Read the model definition and answer for the solid it produces. Units are mm, in the model's axes. A direction names the side the tool comes from. Coordinates: 2 decimals unless noted, no trailing zeros. Write each loop counter-clockwise with the first axis right and the second up, starting at its lowest first coordinate (ties: lowest second). Pieces come first, ordered by that corner, then holes.
(1) The mould has two halves that part along Y. Classify faces 1 (the conical face through (-23.226, 19.757, -0.871)), 2 (the cylindrical face through (-11.668, 34.51, -15.217)), 3 (the flat face through (69, 0, 0)), 4 (the conical face through (163.226, 50.243, 0.871)): +Y half, -Y half, draft (parallel to the pull), parting line (faces both ways), or undercut.
(2) Section A-A on z = 0 is taken. Write down the section's boundary in (x, y) (3 decimals), then the cut area to 3 significant figures.
(3) Which of the six approach directions +Z, -Z, +X, -X, +Y, -Y give full straight-line access (tool end or side, diameter ignored) to faces 5 (the conical face through (163.226, 19.757, 0.871)), 6 (the cylindrical face through (121.28, 34.51, -4.16))?
(4) Find the intervals of material crossed by probe 1 along X at (y, z) = (32, 0) (3 decimals); probe 2 along X at (y, z) = (34.5, -6); probe 3 along X at (y, z) = (32.5, -17.5), in increasing order.
(5) Section C-C on x = 80 is taken. Write down the section's boundary in (y, z), then the cut area to 3 significant figures.
(6) Given pin 1 (2 mm diameter, centred on y = 21, z = 16.5, fed in from +X); pin 2 (20.5 mm diameter, centred on x = 57.5, y = 20.5, fed in from -Z); pin 3 (12 mm diameter, centred on x = 13, y = 57, fed in from +Z); pin 4 (10 mm diameter, centred on x = 31, z = -18.5, fed in from -Y), each flat-ended and moving along its own axis, determine where each tip first touches the part or whether it passes through.
(7) Section B-B on y = 26.5 is taken. Write down the section's boundary in (x, z) (3 decimals), then the cut area to 3 significant figures.
(8) Section D-D on z = -7.5 is taken. State how many separate pieces and enclosed holes the cut face has, then the cut area to 3 significant figures.
from build123d import *

# Parameters (mm, degrees)
SKETCH1_R            = 19.175
BOSS_EXTRUDE1_DEPTH  = 70
SKETCH3_R            = 26
SKETCH3_R_2          = 19.175
BOSS_EXTRUDE2_DEPTH  = 15
FILLET1_R            = 5
CHAMFER2_START       = 15
CHAMFER2_3_OUTLINE_W = 198
CHAMFER2_3_OUTLINE_H = 58
CHAMFER2_3_DEPTH     = 5
CHAMFER1_SIZE        = 1


with BuildPart() as part:
    # Sketch1 → Boss-Extrude1 (new body)
    with BuildSketch(Plane(origin=(0, 0, 0), x_dir=(1, 0, 0), z_dir=(0, 1, 0))):
        with BuildLine():
            Line((19.306734576, -12.5), (120.693265424, -12.5))
            ThreePointArc((120.693265424, -12.5), (129.011369512, -20.205197351), (140, -23))
            ThreePointArc((140, -23), (163, 0), (140, 23))
            ThreePointArc((140, 23), (129.011369512, 20.205197351), (120.693265424, 12.5))
            Line((120.693265424, 12.5), (19.306734576, 12.5))
            ThreePointArc((19.306734576, 12.5), (10.988630488, 20.205197351), (0, 23))
            ThreePointArc((0, 23), (-23, 0), (0, -23))
            ThreePointArc((0, -23), (10.988630488, -20.205197351), (19.306734576, -12.5))
        make_face()
        with Locations(Location((0, 0, 0), (0, 0, 270))):
            Circle(SKETCH1_R, mode=Mode.SUBTRACT)
        with Locations(Location((140, 0, 0), (0, 0, 270))):
            Circle(SKETCH1_R, mode=Mode.SUBTRACT)
    extrude(amount=BOSS_EXTRUDE1_DEPTH)

    # Sketch3 → Boss-Extrude2 (add)
    # profile 1 of 2: a face of its own
    with BuildSketch(Plane.XZ):
        Circle(SKETCH3_R)
        with Locations(Location((0, 0, 0), (0, 0, 90))):
            Circle(SKETCH3_R_2, mode=Mode.SUBTRACT)
    # profile 2 of 2: a face of its own
    with BuildSketch(Plane.XZ):
        with Locations((140, 0)):
            Circle(SKETCH3_R)
        with Locations(Location((140, 0, 0), (0, 0, 90))):
            Circle(SKETCH3_R_2, mode=Mode.SUBTRACT)
    extrude(amount=-BOSS_EXTRUDE2_DEPTH)

    # Fillet1
    fillet1_edges = [part.edges().sort_by_distance(p)[0] for p in [
        (22.79802623, 7.5, -12.5),
        (22.79802623, 7.5, 12.5),
        (117.20197377, 7.5, -12.5),
        (117.20197377, 7.5, 12.5),
    ]]
    fillet(fillet1_edges, radius=FILLET1_R)

    # Chamfer2: read off the stored shape, not the designer's step
    # Chamfer2 outline → Chamfer2 (revolve)
    with BuildSketch(Plane.XY):
        Polygon((28, 15), (23, 20), (23, 15), align=None)
    revolve(axis=Axis((0, 0, 0), (0, 1, 0)))

    # Chamfer2 2 outline → Chamfer2 2 (revolve)
    with BuildSketch(Plane(origin=(140, 0, 0), x_dir=(1, 0, 0), z_dir=(0, 0, 1))):
        Polygon((28, 15), (23, 20), (23, 15), align=None)
    revolve(axis=Axis((140, 0, 0), (0, 1, 0)))

    # Chamfer2 3 outline → Chamfer2 3 (cut)
    with BuildSketch(Plane(origin=(0, 0, 0), x_dir=(1, 0, 0), z_dir=(0, 1, 0)).offset(CHAMFER2_START)):
        with Locations((70, 0)):
            Rectangle(CHAMFER2_3_OUTLINE_W, CHAMFER2_3_OUTLINE_H)
        with BuildLine():
            ThreePointArc((25.588083164, -12.5), (23.254941851, -13.0777323), (21.460972976, -14.677419355))
            ThreePointArc((21.460972976, -14.677419355), (-26, 0), (21.460972976, 14.677419355))
            ThreePointArc((21.460972976, 14.677419355), (23.254941851, 13.0777323), (25.588083164, 12.5))
            Line((25.588083164, 12.5), (114.411916836, 12.5))
            ThreePointArc((114.411916836, 12.5), (116.745058149, 13.0777323), (118.539027024, 14.677419355))
            ThreePointArc((118.539027024, 14.677419355), (166, 0), (118.539027024, -14.677419355))
            ThreePointArc((118.539027024, -14.677419355), (116.745058149, -13.0777323), (114.411916836, -12.5))
            Line((114.411916836, -12.5), (25.588083164, -12.5))
        make_face(mode=Mode.SUBTRACT)
    extrude(amount=CHAMFER2_3_DEPTH, mode=Mode.SUBTRACT)

    # Mirror1: read off the stored shape, not the designer's step
    # Mirror1: part across plane


with BuildPart() as part_1:
    add(part.part)
    add(part.part.mirror(Plane(origin=(0, 35, 0), x_dir=(0, 0, 1), z_dir=(0, -1, 0))))

    # Chamfer1
    chamfer1_edges = [part_1.edges().sort_by_distance(p)[0] for p in [
        (166, 70, 0),
        (70, 70, -12.5),
        (70, 70, 12.5),
        (-26, 70, 0),
        (116.745058149, 70, -13.0777323),
        (116.745058149, 70, 13.0777323),
        (23.254941851, 70, -13.0777323),
        (23.254941851, 70, 13.0777323),
        (70, 0, -12.5),
        (166, 0, 0),
        (70, 0, 12.5),
        (-26, 0, 0),
        (116.745058149, 0, -13.0777323),
        (116.745058149, 0, 13.0777323),
        (23.254941851, 0, -13.0777323),
        (23.254941851, 0, 13.0777323),
    ]]
    chamfer(chamfer1_edges, length=CHAMFER1_SIZE)


solid = part_1.part
Response:
1. face 1: undercut
1. face 2: draft
1. face 3: -Y half
1. face 4: undercut
2. outline: (-26, 1) - (-25, 0) - (-19.175, 0) - (-19.175, 70) - (-25, 70) - (-26, 69) - (-26, 53) - (-23, 50) - (-23, 20) - (-26, 17) - close; (19.175, 0) - (120.825, 0) - (120.825, 70) - (19.175, 70) - close; (159.175, 0) - (165, 0) - (166, 1) - (166, 17) - (163, 20) - (163, 50) - (166, 53) - (166, 69) - (165, 70) - (159.175, 70) - close
2. area: 7,870 mm2
3. face 5: none
3. face 6: +Y, -Y
4. probe 1: x = -23 to -19.175, 19.175 to 120.825, 159.175 to 163
4. probe 2: x = -22.2 to -18.21, 18.21 to 121.79, 158.21 to 162.2
4. probe 3: x = -14.92 to -7.84, 7.84 to 14.92, 125.08 to 132.16, 147.84 to 154.92
5. outline: (0, -11.5) - (1, -12.5) - (69, -12.5) - (70, -11.5) - (70, 11.5) - (69, 12.5) - (1, 12.5) - (0, 11.5) - close
5. area: 1,750 mm2
6. pin 1: stops at x = 156.99
6. pin 2: stops at z = -12.5
6. pin 3: stops at z = 25.04
6. pin 4: passes through
7. outline: (19.307, -12.5) - (120.693, -12.5) arc R23 ccw (long way) to (120.693, 12.5) - (19.307, 12.5) arc R23 ccw (long way) to start; hole circle Ø38.35 at (0, 0); hole circle Ø38.35 at (140, 0)
7. area: 3,420 mm2
8. separate pieces: 3
8. enclosed holes: 0
8. area: 8,130 mm2
